from build123d import *

# Parameters (mm, degrees)
F0_W     = 90
F0_H     = 45
F1_DEPTH = 5
F2_R     = 5
F3_W     = 70
F3_H     = 40
F4_DEPTH = 1
F6_DEPTH = 25
F7_R     = 1.5
F8_DEPTH = 25


with BuildPart() as f1:
    # F0 (on Top) → F1 (new body)
    with BuildSketch(Plane.XY):
        with Locations((45, 22.5)):
            Rectangle(F0_W, F0_H)
    extrude(amount=F1_DEPTH)

    # F2
    f2_edges = [f1.edges().sort_by_distance(p)[0] for p in [
        (90, 45, 2.5),
        (90, 0, 2.5),
        (0, 45, 2.5),
        (0, 0, 2.5),
    ]]
    fillet(f2_edges, radius=F2_R)

    # F3 (on Top) → F4 (cut)
    with BuildSketch(Plane.XY):
        with Locations((45, 25)):
            Rectangle(F3_W, F3_H)
    extrude(amount=F4_DEPTH, mode=Mode.SUBTRACT)

    # F5 (on face) → F6 (cut)
    with BuildSketch(Plane.XY.offset(5)):
        with BuildLine():
            Line((75, 37), (15, 37))
            ThreePointArc((15, 37), (13.585786, 36.414214), (13, 35))
            Line((13, 35), (13, 10))
            ThreePointArc((13, 10), (13.585786, 8.585786), (15, 8))
            Line((15, 8), (75, 8))
            ThreePointArc((75, 8), (76.414214, 8.585786), (77, 10))
            Line((77, 10), (77, 35))
            ThreePointArc((77, 35), (76.414214, 36.414214), (75, 37))
        make_face()
    extrude(amount=-F6_DEPTH, mode=Mode.SUBTRACT)

    # F7 (on face) → F8 (cut)
    with BuildSketch(Plane.XY.offset(5)):
        with Locations((5, 22.5)):
            Circle(F7_R)
        with Locations((85, 22.5)):
            Circle(F7_R)
    extrude(amount=-F8_DEPTH, mode=Mode.SUBTRACT)


solid = f1.part
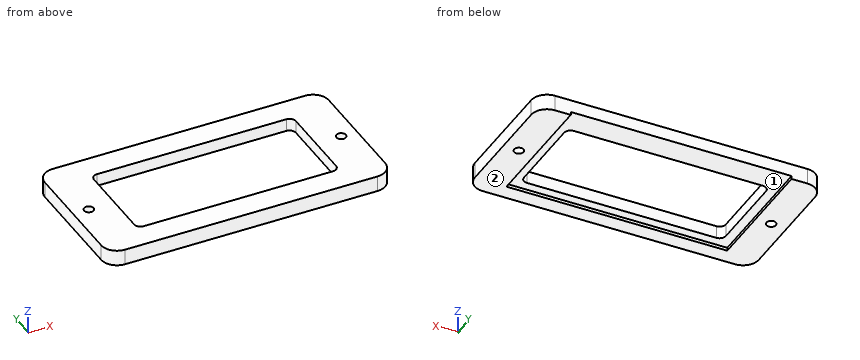
Design review of the part built by this model. Coordinates are the model's own, in mm. Face numbers are marked on the shaded views. Round coordinates to 2 decimals unless told otherwise and drop trailing zeros. Loops run counter-clockwise (first coordinate to the right, second up) from the corner with the lowest first, then second, coordinate; pieces in that order, holes last. Notation, with made-up numbers: (79.25, 84.5) -> (89.25, 84.5) arc R27 ccw to (89.25, 113.5) -> close; hole circle Ø6 at (81.25, -19.5). An arc over 180 degrees is marked (long way). Use one line per item in the form item = value. Start each with the question number.
Q1. We need section C-C on y = 32. Give the boundary of the cut face in (x, z), then the cut area to 3 significant figures.
Q2. Draft analysis for pull direction X (two halves, no side actions). For the marked faces 1 and 2, state which applies: +X half, -X half, draft (parallel to the pull), parting line (faces both ways), or undercut.
Q3. We need section A-A on y = 22.5. Give the boundary of the cut face in (x, z), then the cut area to 3 significant figures.
Q4. Wall thickness on line 1 along Y through (x, z) = (40, 4.4); line 2 along Y through (x, z) = (85, 2.55); line 3 along X through (y, z) = (13.5, 4.65): over which ranges is each line inside the solid? List them lowest first. Write a range as [from, to].
Q5. For pin 1 Ø0.5 at (x, z) = (35.5, 0.5) entering from +Y; pin 2 Ø5 at (x, y) = (5, 22.5) entering from +Z, all flat-tipped, find the tip position at first contact; note any pin that passes through.
Q6. We need section D-D on x = 60.5. Give the boundary of the cut face in (y, z).
Q7. We need section B-B on z = 3.8. Give the boundary of the cut face in (x, y).
Calculated:
q1.outline = (0, 0) -> (10, 0) -> (10, 1) -> (13, 1) -> (13, 5) -> (0, 5) -> close; (77, 1) -> (80, 1) -> (80, 0) -> (90, 0) -> (90, 5) -> (77, 5) -> close
q1.area = 124 mm²
q2.face_1 = undercut
q2.face_2 = draft
q3.outline = (0, 0) -> (3.5, 0) -> (3.5, 5) -> (0, 5) -> close; (6.5, 0) -> (10, 0) -> (10, 1) -> (13, 1) -> (13, 5) -> (6.5, 5) -> close; (77, 1) -> (80, 1) -> (80, 0) -> (83.5, 0) -> (83.5, 5) -> (77, 5) -> close; (86.5, 0) -> (90, 0) -> (90, 5) -> (86.5, 5) -> close
q3.area = 94.0 mm²
q4.line_1 = [0, 8], [37, 45]
q4.line_2 = [0, 21], [24, 45]
q4.line_3 = [0, 13], [77, 90]
q5.pin_1 = 5
q5.pin_2 = 5
q6.outline = (0, 0) -> (5, 0) -> (5, 1) -> (8, 1) -> (8, 5) -> (0, 5) -> close; (37, 1) -> (45, 1) -> (45, 5) -> (37, 5) -> close
q7.outline = (0, 5) arc R5 ccw to (5, 0) -> (85, 0) arc R5 ccw to (90, 5) -> (90, 40) arc R5 ccw to (85, 45) -> (5, 45) arc R5 ccw to (0, 40) -> close; hole circle Ø3 at (5, 22.5); hole (13, 10) arc R2 ccw to (15, 8) -> (75, 8) arc R2 ccw to (77, 10) -> (77, 35) arc R2 ccw to (75, 37) -> (15, 37) arc R2 ccw to (13, 35) -> close; hole circle Ø3 at (85, 22.5)
